Can you work these out from the model? Positions are in its coordinate system, mm. Face numbers are marked on the shaded views. A direction names the side the tool comes from. Round coordinates to 2 decimals unless told otherwise and drop trailing zeros. Loops run counter-clockwise (first coordinate to the right, second up) from the corner with the lowest first, then second, coordinate; pieces in that order, holes last.
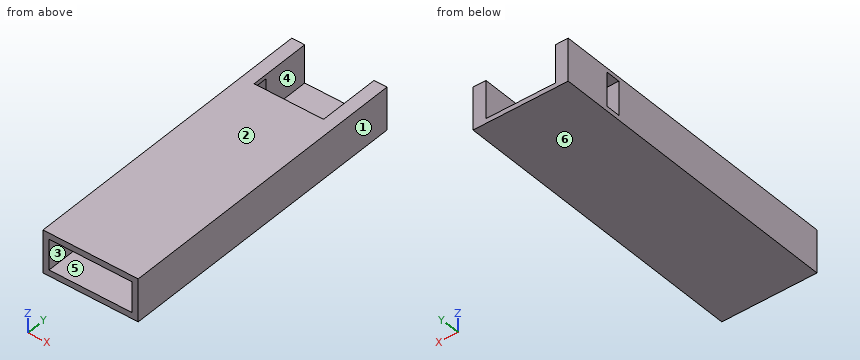
from build123d import *

# Parameters (mm, degrees)
SKETCH1_W           = 31.75
SKETCH1_H           = 14.2875
BOSS_EXTRUDE1_DEPTH = 101.6
SKETCH5_W           = 23.114
SKETCH5_H           = 12.7
CUT_EXTRUDE2_DEPTH  = 20.6375
SKETCH6_W           = 11.345737275
SKETCH6_H           = 4.7625
CUT_EXTRUDE4_DEPTH  = 9.2075
SHELL2_START        = -12.2555
SHELL2_OUTLINE_W    = 0.254
SHELL2_OUTLINE_H    = 11.811
SHELL2_DEPTH        = 10.2235


# Read off the part's stored shape, not the designer's step: Shell2
with BuildPart() as part:
    # Sketch1 → Boss-Extrude1 (new body)
    with BuildSketch(Plane(origin=(0, 0, 0), x_dir=(1, 0, 0), z_dir=(0, 1, 0))):
        with Locations((15.875, 7.14375)):
            Rectangle(SKETCH1_W, SKETCH1_H)
    extrude(amount=BOSS_EXTRUDE1_DEPTH)

    # Sketch5 → Cut-Extrude2 (cut)
    with BuildSketch(Plane(origin=(0, 101.6, 0), x_dir=(1, 0, 0), z_dir=(0, 1, 0))):
        with Locations((15.875, 6.35)):
            Rectangle(SKETCH5_W, SKETCH5_H)
    extrude(amount=-CUT_EXTRUDE2_DEPTH, mode=Mode.SUBTRACT)

    # Sketch6 → Cut-Extrude4 (cut)
    with BuildSketch(Plane.ZY):
        with Locations((-7.027131363, 83.34375)):
            Rectangle(SKETCH6_W, SKETCH6_H)
    extrude(amount=-CUT_EXTRUDE4_DEPTH, mode=Mode.SUBTRACT)

    # Shell2 outline → Shell2 (cut)
    with BuildSketch(Plane.XY.offset(SHELL2_START)):
        Polygon((2.032, 78.9305), (2.032, 0), (29.718, 0), (29.718, 99.568), (29.464, 99.568), (29.464, 78.9305), align=None)
        with Locations((2.159, 93.6625)):
            Rectangle(SHELL2_OUTLINE_W, SHELL2_OUTLINE_H)
    extrude(amount=SHELL2_DEPTH, mode=Mode.SUBTRACT)


solid = part.part
(1) If we section it at B-B, the plane y = 92: List the corners of the cut face in (x, z) for me.
Worked answers:
outline: (0, -14.29) - (31.75, -14.29) - (31.75, 0) - (27.43, 0) - (27.43, -12.7) - (4.32, -12.7) - (4.32, 0) - (0, 0) - close; hole (2.03, -12.26) - (2.29, -12.26) - (2.29, -2.03) - (2.03, -2.03) - close; hole (29.46, -12.26) - (29.72, -12.26) - (29.72, -2.03) - (29.46, -2.03) - close
(2) If I drill on line 1 (X direction, y = 92.5, z = -12); line 2 (Z direction, x = 11.5, y = 6); line 3 (X direction, y = 73.5, z = -5.75), over which ranges is the centre line in solid material (lowest first)?
Worked answers:
line 1: x = 0 to 2.03, 2.29 to 4.32, 27.43 to 29.46, 29.72 to 31.75
line 2: z = -14.29 to -12.26, -2.03 to 0
line 3: x = 0 to 2.03, 29.72 to 31.75
(3) If we section it at C-C, the plane x = 17: List the corners of the cut face in (y, z) for me, then the cut area to 3 significant figures.
Worked answers:
outline: (0, -14.29) - (101.6, -14.29) - (101.6, -12.7) - (80.96, -12.7) - (80.96, 0) - (0, 0) - (0, -2.03) - (78.93, -2.03) - (78.93, -12.26) - (0, -12.26) - close
area: 383 mm2
(4) If we section it at A-A, the plane z = -7.5: State how many separate pieces and enclosed holes the cut face has, then the cut area to 3 significant figures.
Worked answers:
separate pieces: 2
enclosed holes: 1
area: 535 mm2
(5) For the marked faces 4, 5 and 6, which set-ups out of +Z, -Z, +X, -X, +Y, -Y let a thin tool reach every point of the face, with its end or its side?
Worked answers:
face 4: +Z, +Y
face 5: -Y
face 6: -Z, +X, -X, +Y, -Y
(6) Will this pin go through, and if not, where does the flat tip stop? P1, Ø5, axis at x = 14.5, z = -6.5, coming from the -Y side.
Worked answers:
P1: stops at y = 78.93
(7) If we mould it in two halves opening along X, with no side actions, what happens to the marked faces 1, 2 and 3? For each: released by +X, released by -X, zero draft, split by the parting line, or undercut.
Worked answers:
face 1: released by +X
face 2: zero draft
face 3: undercut
(8) If we section it at D-D, the plane y = 15.5: List the corners of the cut face in (x, z) for me.
Worked answers:
outline: (0, -14.29) - (31.75, -14.29) - (31.75, 0) - (0, 0) - close; hole (2.03, -12.26) - (29.72, -12.26) - (29.72, -2.03) - (2.03, -2.03) - close
